```python
from build123d import *

# Parameters (mm, degrees)
F0_W      = 75
F0_H      = 25
F1_DEPTH  = 50
F3_DEPTH  = 50
F5_W      = 75
F5_H      = 40
F6_DEPTH  = 8
F9_R      = 5
F10_R     = 5.3
F11_DEPTH = 2.1


with BuildPart() as f1:
    # F0 (on Top) → F1 (new body)
    with BuildSketch(Plane.XY):
        Rectangle(F0_W, F0_H)
    extrude(amount=F1_DEPTH)


with BuildPart() as f3:
    # F2 (on Right) → F3 (new body, symmetric)
    with BuildSketch(Plane.YZ):
        with BuildLine():
            ThreePointArc((-20, 4.5), (-5.5043109857, 10.5043109857), (0.5, 25))
            ThreePointArc((0.5, 25), (-34.4956890143, 39.4956890143), (-20, 4.5))
        make_face()
    extrude(amount=F3_DEPTH, both=True)


with BuildPart() as f1_1:
    add(f1.part)

    # F4: cut F3
    add(f3.part, mode=Mode.SUBTRACT)


with BuildPart() as f6:
    # F5 (on Top) → F6 (new body)
    with BuildSketch(Plane.XY):
        Rectangle(F5_W, F5_H)
    extrude(amount=F6_DEPTH)


with BuildPart() as f6_1:
    # F7: moved
    add(f6.part.moved(Location((0, 7.5, -8))))

    # F8: union F1
    add(f1_1.part)

    # F9
    f9_edges = [f6_1.edges().sort_by_distance(p)[0] for p in [
        (37.5, -12.5, -1.039392),
        (-37.5, -12.5, -1.039392),
        (37.5, 27.5, -4),
        (-37.5, 27.5, -4),
    ]]
    fillet(f9_edges, radius=F9_R)


with BuildPart() as f11:
    # F10 (on Front) → F11 (new body)
    with BuildSketch(Plane.XZ):
        with Locations((-20, 26)):
            Circle(F10_R)
    extrude(amount=F11_DEPTH)


with BuildPart() as f11_1:
    # F12: moved
    add(f11.part.moved(Location((0, 12.5, 0))))


with BuildPart() as f13_1:
    # F13: instance of F11
    add(f11_1.part.mirror(Plane.YZ))


with BuildPart() as f6_2:
    add(f6_1.part)

    # F14: cut F11, F13_1
    add(f11_1.part, mode=Mode.SUBTRACT)
    add(f13_1.part, mode=Mode.SUBTRACT)


solid = f6_2.part
```
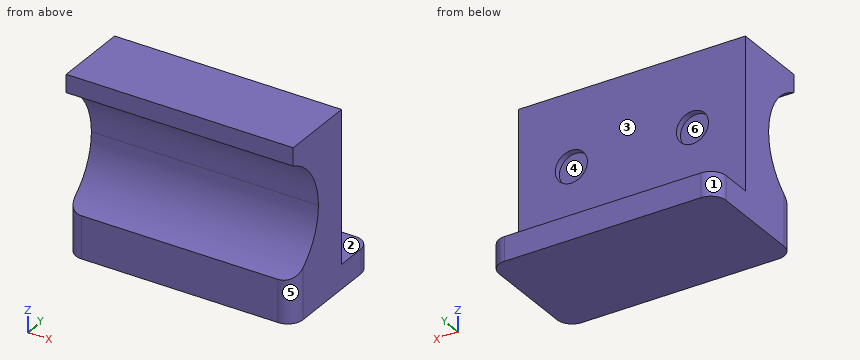
Build history of the part. All positions in model axes, mm. Face numbers are marked on the shaded views. A direction names the side the tool comes from. Coordinates: 2 decimals unless noted, no trailing zeros. Order: outer loops, then holes, each group sorted by start corner. A loop starts at its lowest first (then second) coordinate and runs counter-clockwise, first axis right, second up.
Item 1: Tool access for the marked faces 1 and 2: list every direction of +Z, -Z, +X, -X, +Y, -Y with a clear straight run to the whole face (end or side of a thin tool).
Filled in:
face 1: +Z, -Z, -X, +Y
face 2: +Z, +X, -X, +Y
Item 2: Saw through at C-C on x = 10. List the corners of the cut face in (y, z).
Filled in:
outline: (-12.5, -8) - (27.5, -8) - (27.5, 0) - (12.5, 0) - (12.5, 50) - (-12.5, 50) - (-12.5, 44.08) arc R20.5 cw to (-12.5, 5.92) - close
Item 3: Saw through at D-D on y = 24. List the corners of the cut face in (x, z).
Filled in:
outline: (-37.27, -8) - (37.27, -8) - (37.27, 0) - (-37.27, 0) - close
Item 4: Drop flat-ended pins along their axis: pin 1 Ø8.5 at (x, z) = (-21, 25) entering from +Y; pin 2 Ø5 at (x, z) = (29, 33) entering from -Y; pin 3 Ø5 at (x, z) = (-4.5, 9.5) entering from -Y. Give the stop position or say it passes through.
Filled in:
pin 1: stops at y = 12.5
pin 2: stops at y = -2.39
pin 3: stops at y = -10.19
Item 5: Saw through at B-B on z = 29.5. List the corners of the cut face in (x, y), then the cut area to 3 significant figures.
Filled in:
outline: (-37.5, 0) - (37.5, 0) - (37.5, 12.5) - (23.98, 12.5) - (23.98, 10.4) - (16.02, 10.4) - (16.02, 12.5) - (-16.02, 12.5) - (-16.02, 10.4) - (-23.98, 10.4) - (-23.98, 12.5) - (-37.5, 12.5) - close
area: 904 mm2
Item 6: Drill centre lines: L1, parallel to Z at x = 20, y = 11.1; L2, parallel to Z at x = 29.5, y = 16.5; L3, parallel to Y at x = 24.5, z = 46. Where is each one in solid material? Low to high.
Filled in:
L1: z = -8 to 20.7, 31.3 to 50
L2: z = -8 to 0
L3: y = -12.5 to 12.5
Item 7: Saw through at A-A on x = 20. List the corners of the cut face in (y, z).
Filled in:
outline: (-12.5, -8) - (27.5, -8) - (27.5, 0) - (12.5, 0) - (12.5, 20.7) - (10.4, 20.7) - (10.4, 31.3) - (12.5, 31.3) - (12.5, 50) - (-12.5, 50) - (-12.5, 44.08) arc R20.5 cw to (-12.5, 5.92) - close
Item 8: Mould opens along X. For the marked faces 3, 4, 5 and 6 say: released by +X, released by -X, zero draft, split by the parting line, or undercut.
Filled in:
face 3: zero draft
face 4: undercut
face 5: released by +X
face 6: undercut
